Could you check a few things on this model? Use its own coordinates, in mm. A direction names the side the tool comes from. Give positions to 0.01 mm unless a question says otherwise; leave off trailing zeros. Order: outer loops, then holes, each group sorted by start corner. A loop starts at its lowest first (then second) coordinate and runs counter-clockwise, first axis right, second up. Notation, with made-up numbers: M -9,55 L 45,55 A19 cw 45,91 Z; hole C 15,27.25 d6. An arc over 180 degrees is marked long. Return JSON: item names as keys, results as strings. Group by question number.
```python
from build123d import *

# Parameters (mm, degrees)
F1_DEPTH  = 104.5
F3_DEPTH  = 127.001
F4_W      = 127
F4_H      = 62
F5_DEPTH  = 27
F7_DEPTH  = 93.5104
F8_W      = 78.298144
F8_H      = 207.146659
F9_DEPTH  = 127.001
F11_DEPTH = 63.827166
F12_R     = 12.802334
F12_R_2   = 12.940418
F12_R_3   = 12.784861
F12_R_4   = 13.089145
F13_DEPTH = 25.4


with BuildPart() as f1:
    # F0 (on Front) → F1 (new body)
    with BuildSketch(Plane.XZ):
        with BuildLine():
            ThreePointArc((0, 62.5094), (-35.443943, 54.198998), (-63.5, 31))
            Line((-63.5, 31), (0, 31))
            Line((0, 31), (0, 62.5094))
        make_face()
        Polygon((0, 31), (-63.5, 31), (-63.5, -31), (0, -31), (0, 0), align=None)
        with BuildLine():
            Line((0, 62.5094), (0, 31))
            Line((0, 31), (63.5, 31))
            ThreePointArc((63.5, 31), (35.443943, 54.198998), (0, 62.5094))
        make_face()
        Polygon((63.5, 31), (0, 31), (0, 0), (0, -31), (63.5, -31), align=None)
        with BuildLine():
            Line((0, -31), (-63.5, -31))
            ThreePointArc((-63.5, -31), (-35.441854, -54.192308), (0, -62.5))
            Line((0, -62.5), (0, -31))
        make_face()
        with BuildLine():
            Line((63.5, -31), (0, -31))
            Line((0, -31), (0, -62.5))
            ThreePointArc((0, -62.5), (35.441854, -54.192308), (63.5, -31))
        make_face()
    extrude(amount=F1_DEPTH)

    # F2 (on face) → F3 (cut, through all)
    with BuildSketch(Plane.YZ.offset(63.5)):
        Polygon((-104.5, 72.844587), (-104.5, 31), (-62.5, 64.333223), align=None)
        Polygon((-62.5, -65.093011), (-104.5, -31), (-104.5, -67.313612), align=None)
    extrude(amount=-F3_DEPTH, mode=Mode.SUBTRACT)

    # F4 (on face) → F5 (join)
    with BuildSketch(Plane.XZ.offset(104.5)):
        Rectangle(F4_W, F4_H)
    extrude(amount=F5_DEPTH)

    # F6 (on face) → F7 (cut, through all)
    with BuildSketch(Plane(origin=(0, 0, -31), x_dir=(1, 0, 0), z_dir=(0, 0, -1))):
        with BuildLine():
            ThreePointArc((-63.5, 104.5), (-34.500906, 124.469723), (0, 131.5))
            Line((0, 131.5), (-63.5, 131.5))
            Line((-63.5, 131.5), (-63.5, 104.5))
        make_face()
        with BuildLine():
            ThreePointArc((0, 131.5), (34.500906, 124.469723), (63.5, 104.5))
            Line((63.5, 104.5), (63.5, 131.5))
            Line((63.5, 131.5), (0, 131.5))
        make_face()
    extrude(amount=-F7_DEPTH, mode=Mode.SUBTRACT)

    # F8 (on face) → F9 (cut, through all)
    with BuildSketch(Plane.YZ.offset(63.5)):
        with Locations((-102.975238, -5.202033)):
            Rectangle(F8_W, F8_H)
    extrude(amount=-F9_DEPTH, mode=Mode.SUBTRACT)

    # F10 (on face) → F11 (cut, through all)
    with BuildSketch(Plane.XZ.offset(63.826166)):
        with BuildLine():
            ThreePointArc((53.975, -25.529381), (52.580096, -22.161785), (49.2125, -20.766881))
            Line((49.2125, -20.766881), (49.2125, -25.529381))
            Line((49.2125, -25.529381), (44.45, -25.529381))
            ThreePointArc((44.45, -25.529381), (49.2125, -30.291881), (53.975, -25.529381))
        make_face()
        with BuildLine():
            Line((49.2125, -25.529381), (49.2125, -20.766881))
            ThreePointArc((49.2125, -20.766881), (45.844904, -22.161785), (44.45, -25.529381))
            Line((44.45, -25.529381), (49.2125, -25.529381))
        make_face()
        with BuildLine():
            Line((-49.2125, -25.529381), (-49.2125, -20.766881))
            ThreePointArc((-49.2125, -20.766881), (-52.580096, -28.896977), (-44.45, -25.529381))
            Line((-44.45, -25.529381), (-49.2125, -25.529381))
        make_face()
        with BuildLine():
            ThreePointArc((-44.45, -25.529381), (-45.844904, -22.161785), (-49.2125, -20.766881))
            Line((-49.2125, -20.766881), (-49.2125, -25.529381))
            Line((-49.2125, -25.529381), (-44.45, -25.529381))
        make_face()
        with BuildLine():
            ThreePointArc((-44.45, 25.295729), (-52.580096, 28.663325), (-49.2125, 20.533229))
            Line((-49.2125, 20.533229), (-49.2125, 25.295729))
            Line((-49.2125, 25.295729), (-44.45, 25.295729))
        make_face()
        with BuildLine():
            Line((-49.2125, 25.295729), (-49.2125, 20.533229))
            ThreePointArc((-49.2125, 20.533229), (-45.844904, 21.928133), (-44.45, 25.295729))
            Line((-44.45, 25.295729), (-49.2125, 25.295729))
        make_face()
        with BuildLine():
            ThreePointArc((44.45, 25.295729), (45.844904, 21.928133), (49.2125, 20.533229))
            Line((49.2125, 20.533229), (49.2125, 25.295729))
            Line((49.2125, 25.295729), (44.45, 25.295729))
        make_face()
        with BuildLine():
            Line((49.2125, 25.295729), (49.2125, 20.533229))
            ThreePointArc((49.2125, 20.533229), (52.580096, 21.928133), (53.975, 25.295729))
            ThreePointArc((53.975, 25.295729), (49.2125, 30.058229), (44.45, 25.295729))
            Line((44.45, 25.295729), (49.2125, 25.295729))
        make_face()
    extrude(amount=-F11_DEPTH, mode=Mode.SUBTRACT)

    # F12 (on face) → F13 (cut)
    with BuildSketch(Plane.XZ.offset(63.826166)):
        with Locations((49.2125, -25.529381)):
            Circle(F12_R)
        with Locations((-49.2125, -25.529381)):
            Circle(F12_R_2)
        with Locations((-49.2125, 25.295729)):
            Circle(F12_R_3)
        with Locations((49.2125, 25.295729)):
            Circle(F12_R_4)
    extrude(amount=-F13_DEPTH, mode=Mode.SUBTRACT)


solid = f1.part
```
1. Imagine slicing it at A-A, the plane y = -26. Count the separate pieces of the cut face and the enclosed holes in it, plus the area to 3 significant figures.
2. If we mould it in two halves opening along X, with no side actions, what happens to faces 1 (the flat face through (-1, 0, 1)), 2 (the cylindrical face through (-59.36, -51.3, 17.52)), 3 (the flat face through (63.5, -31, 0)), 4 (the cylindrical face through (36.423, -51.304, -24.966))? For each: pulls with the +X half, pulls with the -X half, needs draft (parallel to the pull), parting line crosses it, or undercut.
3. Imagine slicing it at C-C, the plane y = -48.5. Please give me the cut outline in (x, z), plus the area to 3 significant figures.
4. Imagine slicing it at B-B, the plane z = -22.5. Please give me the cut outline in (x, y), plus the area to 3 significant figures.
5. Which directions (+Z, -Z, +X, -X, +Y, -Y) give clear straight access to the entire face, cutting with the end or side of a thin tool? Please do faces 5 (the flat face through (-63.5, -31, 0)), 6 (the flat face through (-49, -38.426, -31)).
6. For pin 1 (15.5 mm diameter, centred on x = 49.21, z = -25.53, fed in from -Y); pin 2 (12 mm diameter, centred on x = -25, y = -44.5, fed in from +Z); pin 3 (4 mm diameter, centred on x = -35.5, y = -39, fed in from +Z), each with a flat end and sliding along its axis, tell me the tip position at first contact or that it passes through.
7. I need wall thicknesses on L1, parallel to Z at x = -52.5, y = -54; L2, parallel to Z at x = -40, y = -50; L3, parallel to X at y = -51, z = 29. Which ranges of each line are inside material? Lowest first, please. Write a range as from..to.
8. Imagine slicing it at D-D, the plane z = 17.5. Please give me the cut outline in (x, y), plus the area to 3 significant figures.
Values:
{
 "1": {"separate pieces": "1", "enclosed holes": "4", "area": "13,200 mm²"},
 "2": {"face 1": "needs draft", "face 2": "undercut", "face 3": "pulls with the +X half", "face 4": "undercut"},
 "3": {"outline": "M -63.5,-31 A79.75 ccw 0,-62.5 A79.75 ccw 63.5,-31 L 63.5,31 A79.74 ccw 0,62.51 A79.74 ccw -63.5,31 Z; hole C -49.21,-25.53 d25.88; hole C -49.21,25.3 d25.57; hole C 49.21,25.3 d26.18; hole C 49.21,-25.53 d25.6", "area": "11,400 mm²"},
 "4": {"outline": "M -63.5,-63.83 L -61.79,-63.83 L -61.79,-38.43 L -52.89,-38.43 L -52.89,0 L -63.5,0 Z; M -45.54,-38.43 L -36.63,-38.43 L -36.63,-63.83 L 36.77,-63.83 L 36.77,-38.43 L 45.54,-38.43 L 45.54,0 L -45.54,0 Z; M 52.89,-38.43 L 61.65,-38.43 L 61.65,-63.83 L 63.5,-63.83 L 63.5,0 L 52.89,0 Z", "area": "6,270 mm²"},
 "5": {"face 5": "+Z, -Z, -X, +Y, -Y", "face 6": "-Y"},
 "6": {"pin 1": "stops at y = -38.43", "pin 2": "stops at z = 60.21", "pin 3": "stops at z = 55.13"},
 "7": {"L1": "z = -42.78..-38.05, -13.01..12.94, 37.65..42.79", "L2": "z = -51.74..-34.62, -16.44..16.43, 34.16..51.75", "L3": "x = -63.5..-61.45, -36.98..36.66, 61.77..63.5"},
 "8": {"outline": "M -63.5,-63.83 L -59.35,-63.83 L -59.35,-38.43 L -39.08,-38.43 L -39.08,-63.83 L 38.7,-63.83 L 38.7,-38.43 L 59.73,-38.43 L 59.73,-63.83 L 63.5,-63.83 L 63.5,0 L -63.5,0 Z", "area": "7,060 mm²"}
}
